Design review of the part built by this model. Coordinates are the model's own, in mm. Give positions to 0.01 mm unless a question says otherwise; leave off trailing zeros. Order: outer loops, then holes, each group sorted by start corner. A loop starts at its lowest first (then second) coordinate and runs counter-clockwise, first axis right, second up. Notation, with made-up numbers: M 77.25,20 L 128.25,20 A19 ccw 128.25,36 Z; hole C 47,33 d2. An arc over 180 degrees is marked long. Answer as a JSON object with one key per item and string values.
from build123d import *

# Parameters (mm, degrees)
F0_W     = 80
F0_H     = 20
F1_DEPTH = 5
F2_R     = 5
F3_DEPTH = 5.001
F4_R     = 5


with BuildPart() as f1:
    # F0 (on Top) → F1 (new body)
    with BuildSketch(Plane.XY):
        Rectangle(F0_W, F0_H)
    extrude(amount=F1_DEPTH)

    # F2 (on Top) → F3 (cut, through all)
    with BuildSketch(Plane.XY):
        with Locations((-30.004952, 0)):
            Circle(F2_R)
        with Locations((27.362093, 0)):
            Circle(F2_R)
    extrude(amount=F3_DEPTH, mode=Mode.SUBTRACT)

    # F4
    f4_edges = [f1.edges().sort_by_distance(p)[0] for p in [
        (40, -10, 2.5),
        (40, 10, 2.5),
        (-40, -10, 2.5),
        (-40, 10, 2.5),
    ]]
    fillet(f4_edges, radius=F4_R)


solid = f1.part
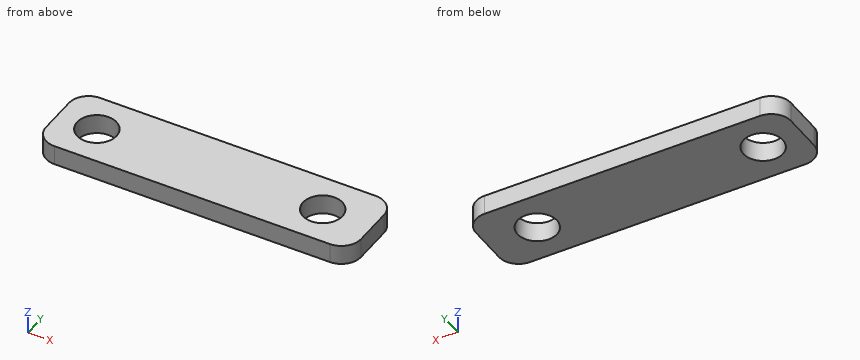
(1) We need section C-C (y = 7.75). Write out the cut boundary in (x, z), plus the area to 3 significant figures.
Checked values:
{"outline": "M -39.18,0 L 39.18,0 L 39.18,5 L -39.18,5 Z", "area": "392 mm^2"}
(2) Insertion check: pin 1 (10 mm diameter, centred on x = 17, y = -5.5, fed in from -Z). The pin has a flat end and moves straight along its axis. Give the tip position at first contact, or say it passes through.
Checked values:
{"pin 1": "stops at z = 0"}
(3) We need section D-D (y = -7.5). Write out the cut boundary in (x, z), plus the area to 3 significant figures.
Checked values:
{"outline": "M -39.33,0 L 39.33,0 L 39.33,5 L -39.33,5 Z", "area": "393 mm^2"}
(4) To check wall thickness, follow L1, parallel to X at y = 0, z = 3.6; L2, parallel to Y at x = 30, z = 1.7; L3, parallel to X at y = -1.75, z = 1.2. State the ranges of each line that lie inside material, in increasing order. Write a range as from..to.
Checked values:
{"L1": "x = -40..-35, -25..22.36, 32.36..40", "L2": "y = -10..-4.25, 4.25..10", "L3": "x = -40..-34.69, -25.32..22.68, 32.05..40"}
(5) We need section A-A (y = 0). Write out the cut boundary in (x, z), plus the area to 3 significant figures.
Checked values:
{"outline": "M -40,0 L -35,0 L -35,5 L -40,5 Z; M -25,0 L 22.36,0 L 22.36,5 L -25,5 Z; M 32.36,0 L 40,0 L 40,5 L 32.36,5 Z", "area": "300 mm^2"}
(6) We need section B-B (z = 2.4). Write out the cut boundary in (x, y).
Checked values:
{"outline": "M -40,-5 A5 ccw -35,-10 L 35,-10 A5 ccw 40,-5 L 40,5 A5 ccw 35,10 L -35,10 A5 ccw -40,5 Z; hole C -30,0 d10; hole C 27.36,0 d10"}
